```python
from build123d import *

# Parameters (mm, degrees)
SKETCH1_W           = 27.998507133
SKETCH1_H           = 69.998003006
SKETCH1_R           = 2.078999996
SKETCH1_R_2         = 3.125
SKETCH1_R_3         = 2.078894146
BOSS_EXTRUDE1_DEPTH = 5.8
CUT_EXTRUDE1_DEPTH  = 5.1
FILLET1_R           = 2


with BuildPart() as part:
    # Sketch1 → Boss-Extrude1 (new body)
    with BuildSketch(Plane.XY):
        with Locations((0.000746433, -0.000998497)):
            Rectangle(SKETCH1_W, SKETCH1_H)
        with Locations((0.000493893, -21.295000553)):
            Circle(SKETCH1_R, mode=Mode.SUBTRACT)
        with Locations((0, 3.703561495)):
            Circle(SKETCH1_R_2, mode=Mode.SUBTRACT)
        with Locations((0.000493654, 28.705001831)):
            Circle(SKETCH1_R_3, mode=Mode.SUBTRACT)
    extrude(amount=BOSS_EXTRUDE1_DEPTH)

    # Sketch2 → Cut-Extrude1 (cut)
    with BuildSketch(Plane(origin=(0, 0, 0), x_dir=(-1, 0, 0), z_dir=(0, 0, -1))):
        Polygon((2.928753578, 8.776311495), (-2.928753578, 8.776311495), (-5.857507156, 3.703561495), (-2.928753578, -1.369188505), (2.928753578, -1.369188505), (5.857507156, 3.703561495), align=None)
    extrude(amount=-CUT_EXTRUDE1_DEPTH, mode=Mode.SUBTRACT)

    # Fillet1
    fillet1_edges = [part.edges().sort_by_distance(p)[0] for p in [
        (-13.998507133, 34.998003006, 2.9),
        (14, 34.998003006, 2.9),
        (14, -35, 2.9),
        (-13.998507133, -35, 2.9),
    ]]
    fillet(fillet1_edges, radius=FILLET1_R)


solid = part.part
```
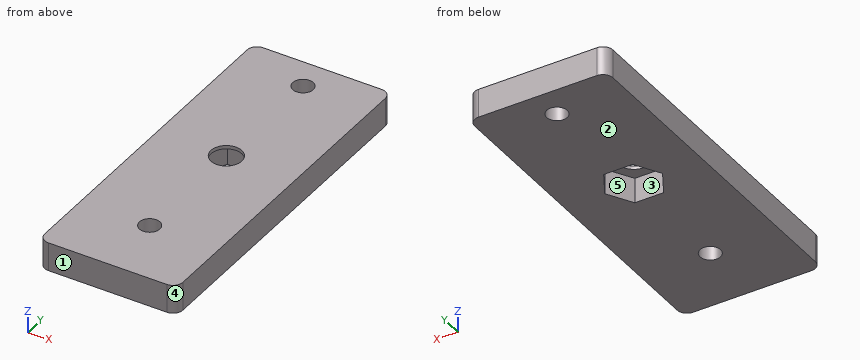
The model under review builds one solid part; all positions refer to its coordinate system, in mm. Face numbers are marked on the shaded views. A direction names the side the tool comes from. Coordinates: 2 decimals unless noted, no trailing zeros. Write each loop counter-clockwise with the first axis right and the second up, starting at its lowest first coordinate (ties: lowest second). Pieces come first, ordered by that corner, then holes. Notation, with made-up numbers: (81.25, 6) - (115.25, 6) arc R25 ccw to (115.25, 29) - close; hole circle Ø11 at (-17.75, 62). An arc over 180 degrees is marked (long way). Answer in a Markdown table with one row per item. Add a question column.
Q1. Clearance check with flat-ended pins moving along their axes: pin 1 (2.5 mm diameter, centred on x = 0, y = -21.3, fed in from +Z); pin 2 (7 mm diameter, centred on x = 0, y = 3.7, fed in from -Z). State where each tip first meets the part, or that it passes through.
Q2. To check wall thickness, follow line 1 along Y through (x, z) = (-0.25, 1.7); line 2 along Y through (x, z) = (0, 5.6); line 3 along Y through (x, z) = (5.75, 2.55). State the ranges of each line that lie inside material, in increasing order. Write a range as from..to.
Q3. For the marked faces 4 and 5, list the 3-axis set-ups (+Z, -Z, +X, -X, +Y, -Y) from which the entire face can be reached by the end or side of a thin tool; tool diameter is ignored.
Q4. Draft analysis for pull direction Y (two halves, no side actions). For the marked faces 1, 2 and 3, state which applies: +Y half, -Y half, draft (parallel to the pull), parting line (faces both ways), or undercut.
Q5. Consider section B-B on z = 4.3. Give the boundary of the cut face in (x, y) (1 decimal).
Q6. Consider section A-A on x = 0. Give the boundary of the cut face in (y, z), then the cut area to 3 significant figures.
Answers below:
| question | item | result |
|---|---|---|
| 1 | pin 1 | through |
| 1 | pin 2 | z = 5.1 |
| 2 | line 1 | -35..-23.36, -19.23..-1.37, 8.78..26.64, 30.77..35 |
| 2 | line 2 | -35..-23.37, -19.22..0.58, 6.83..26.63, 30.78..35 |
| 2 | line 3 | -35..3.52, 3.89..35 |
| 3 | face 4 | +Z, -Z, +X, -Y |
| 3 | face 5 | -Z |
| 4 | face 1 | -Y half |
| 4 | face 2 | draft |
| 4 | face 3 | undercut |
| 5 | outline | (-14, -33) arc R2 ccw to (-12, -35) - (12, -35) arc R2 ccw to (14, -33) - (14, 33) arc R2 ccw to (12, 35) - (-12, 35) arc R2 ccw to (-14, 33) - close; hole (-5.9, 3.7) - (-2.9, -1.4) - (2.9, -1.4) - (5.9, 3.7) - (2.9, 8.8) - (-2.9, 8.8) - close; hole circle Ø4.2 at (0, -21.3); hole circle Ø4.2 at (0, 28.7) |
| 6 | outline | (-35, 0) - (-23.37, 0) - (-23.37, 5.8) - (-35, 5.8) - close; (-19.22, 0) - (-1.37, 0) - (-1.37, 5.1) - (0.58, 5.1) - (0.58, 5.8) - (-19.22, 5.8) - close; (6.83, 5.1) - (8.78, 5.1) - (8.78, 0) - (26.63, 0) - (26.63, 5.8) - (6.83, 5.8) - close; (30.78, 0) - (35, 0) - (35, 5.8) - (30.78, 5.8) - close |
| 6 | area | 302 mm² |
